from build123d import *

# Parameters (mm, degrees)
SKETCH1_W                              = 110.475
SKETCH1_H                              = 90
SKETCH1_W_2                            = 100.475
SKETCH1_H_2                            = 80
SKETCH1_W_3                            = 5
BOSS_EXTRUDE1_DEPTH                    = 20
CBORE_FOR_M4_SBHCS1_AT_2_COUNT         = 2
CBORE_FOR_M4_SBHCS1_AT_2_PITCH         = 40
CBORE_FOR_M5_HEX_HEAD_BOLT1_AT_2_COUNT = 2
CBORE_FOR_M5_HEX_HEAD_BOLT1_AT_2_PITCH = 50
SKETCH7_W                              = 5
SKETCH7_H                              = 80
CUT_EXTRUDE1_DEPTH                     = 30


with BuildPart() as part:
    # Sketch1 → Boss-Extrude1 (new body)
    # profile 1 of 2: a face of its own
    with BuildSketch(Plane(origin=(0, 0, 0), x_dir=(0, 0, -1), z_dir=(1, 0, 0))):
        Rectangle(SKETCH1_W, SKETCH1_H)
        Rectangle(SKETCH1_W_2, SKETCH1_H_2, mode=Mode.SUBTRACT)
    # profile 2 of 2: a face of its own
    with BuildSketch(Plane(origin=(0, 0, 0), x_dir=(0, 0, -1), z_dir=(1, 0, 0))):
        with Locations((22.7375, 0)):
            Rectangle(SKETCH1_W_3, SKETCH1_H_2)
    extrude(amount=BOSS_EXTRUDE1_DEPTH)

    # Sketch3 → CBORE for M4 SBHCS1 (revolve, cut)
    with BuildSketch(Plane(origin=(10, -40, -23.4125), x_dir=(0, 0, 1), z_dir=(1, 0, 0))):
        Polygon((0, 0), (0, 9.151936393), (2.25, 7.8), (2.25, 2.2), (5, 2.2), (5, 0), align=None)
    cbore_for_m4_sbhcs1 = revolve(axis=Axis((10, -33.65, -23.4125), (0, -1, 0)), mode=Mode.SUBTRACT)

    # CBORE for M4 SBHCS1 at 2: CBORE for M4 SBHCS1 ×2
    with Locations(*[(0, 0, i * CBORE_FOR_M4_SBHCS1_AT_2_PITCH) for i in range(1, CBORE_FOR_M4_SBHCS1_AT_2_COUNT)]):
        add(cbore_for_m4_sbhcs1, mode=Mode.SUBTRACT)

    # Sketch6 → CBORE for M5 Hex Head Bolt1 (revolve, cut)
    with BuildSketch(Plane(origin=(10, 30, 55.2375), x_dir=(0, -1, 0), z_dir=(1, 0, 0))):
        Polygon((0, 0), (0, 11.451936393), (2.25, 10.1), (2.25, 4.2), (2.5, 4.2), (2.5, 0), align=None)
    cbore_for_m5_hex_head_bolt1 = revolve(axis=Axis((10, 30, 61.5875), (0, 0, -1)), mode=Mode.SUBTRACT)

    # CBORE for M5 Hex Head Bolt1 at 2: CBORE for M5 Hex Head Bolt1 ×2
    with Locations(*[(0, -i * CBORE_FOR_M5_HEX_HEAD_BOLT1_AT_2_PITCH, 0) for i in range(1, CBORE_FOR_M5_HEX_HEAD_BOLT1_AT_2_COUNT)]):
        add(cbore_for_m5_hex_head_bolt1, mode=Mode.SUBTRACT)

    # Mirror1: CBORE for M5 Hex Head Bolt1 across plane
    add(cbore_for_m5_hex_head_bolt1.mirror(Plane.XY), mode=Mode.SUBTRACT)

    # Mirror1 copy 1 sketch → Mirror1 copy 1 (revolve, cut)
    with BuildSketch(Plane(origin=(10, -20, -55.2375), x_dir=(0, -1, 0), z_dir=(1, 0, 0))):
        Polygon((0, 0), (0, -11.451936393), (2.25, -10.1), (2.25, -4.2), (2.5, -4.2), (2.5, 0), align=None)
    revolve(axis=Axis((10, -20, -61.5875), (0, 0, -1)), mode=Mode.SUBTRACT)

    # Sketch7 → Cut-Extrude1 (cut)
    with BuildSketch(Plane.ZY):
        with Locations((-22.7375, 0)):
            Rectangle(SKETCH7_W, SKETCH7_H)
    extrude(amount=-CUT_EXTRUDE1_DEPTH, mode=Mode.SUBTRACT)


solid = part.part
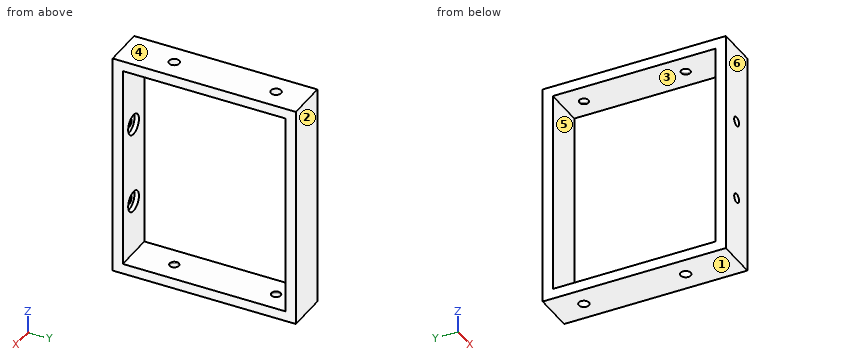
Here's how the part is built. I have some questions about the finished solid (model axes, mm). Face numbers are marked on the shaded views. A direction names the side the tool comes from. Round coordinates to 2 decimals unless told otherwise and drop trailing zeros. Order: outer loops, then holes, each group sorted by start corner. A loop starts at its lowest first (then second) coordinate and runs counter-clockwise, first axis right, second up. Notation, with made-up numbers: M 16,9 L 38,9 A33 cw 38,44 Z; hole C -11.75,13.25 d2. An arc over 180 degrees is marked long. One line per question, with ' | ' between items.
1) We'd pull the mould along Z, two halves only. Please class the marked faces 1, 2, 3 and 4: released by +Z, released by -Z, zero draft, split by the parting line, or undercut.
Checked values:
face 1: released by -Z | face 2: zero draft | face 3: undercut | face 4: released by +Z
2) I need wall thicknesses on line 1 (Y direction, x = 10, z = -54.1); line 2 (Y direction, x = 10, z = 50.7); line 3 (Z direction, x = 10, y = -40.65). Which ranges of each line are inside material? Lowest first, please.
Checked values:
line 1: y = -45 to -22.5, -17.5 to 27.5, 32.5 to 45 | line 2: y = -45 to -22.25, -17.75 to 27.75, 32.25 to 45 | line 3: z = -55.24 to -28.41, -18.41 to 11.59, 21.59 to 55.24
3) Imagine slicing it at A-A, the plane y = 35.5. Write out the boundary of the cut face in (x, z).
Checked values:
outline: M 0,-55.24 L 20,-55.24 L 20,-50.24 L 0,-50.24 Z; M 0,50.24 L 20,50.24 L 20,55.24 L 0,55.24 Z
4) On a 3-axis mill with a long thin cutter (end or side, diameter ignored), from which of +Z, -Z, +X, -X, +Y, -Y can I reach the whole of each face in a straight line? I mean the marked faces 5 and 6. Say none if no direction works.
Checked values:
face 5: +X, -X | face 6: +Z, -Z, +X, -X, -Y
5) Imagine slicing it at C-C, the plane z = 28. Write out the boundary of the cut face in (x, y), plus the area to 3 significant figures.
Checked values:
outline: M 0,-45 L 20,-45 L 20,-40 L 0,-40 Z; M 0,40 L 20,40 L 20,45 L 0,45 Z | area: 200 mm²
6) Imagine slicing it at B-B, the plane x = 1.5. Write out the boundary of the cut face in (y, z).
Checked values:
outline: M -45,-55.24 L 45,-55.24 L 45,55.24 L -45,55.24 Z; hole M -40,-50.24 L 40,-50.24 L 40,50.24 L -40,50.24 Z
7) Imagine slicing it at D-D, the plane x = 10. Count the separate pieces of the cut face and the enclosed holes in it, plus the area to 3 significant figures.
Checked values:
separate pieces: 6 | enclosed holes: 0 | area: 1,740 mm²
